from build123d import *

# Parameters (mm, degrees)
SALIENTE_EXTRUIR1_DEPTH = 1.5
CROQUIS2_W              = 25
CROQUIS2_H              = 3.1
CORTAR_EXTRUIR1_DEPTH   = 10


with BuildPart() as part:
    # Croquis1 → Saliente-Extruir1 (new, symmetric)
    with BuildSketch(Plane.XY):
        Polygon((-31.9, -27), (-31.9, -45), (-21, -45), (-21, -41.9), (-7, -41.9), (-7, -45), (7, -45), (7, -41.9), (21, -41.9), (21, -45), (31.9, -45), (31.9, -27), (35, -27), (35, -9), (31.9, -9), (31.9, 9), (35, 9), (35, 27), (31.9, 27), (31.9, 45), (21, 45), (21, 41.9), (7, 41.9), (7, 45), (-7, 45), (-7, 41.9), (-21, 41.9), (-21, 45), (-31.9, 45), (-31.9, 27), (-35, 27), (-35, 9), (-31.9, 9), (-31.9, -9), (-35, -9), (-35, -27), align=None)
    extrude(amount=SALIENTE_EXTRUIR1_DEPTH, both=True)

    # Croquis2 → Cortar-Extruir1 (cut)
    with BuildSketch(Plane(origin=(0, 0, -1.5), x_dir=(-1, 0, 0), z_dir=(0, 0, -1))):
        with Locations((0, -25.45)):
            Rectangle(CROQUIS2_W, CROQUIS2_H)
    extrude(amount=-CORTAR_EXTRUIR1_DEPTH, mode=Mode.SUBTRACT)


solid = part.part
Input: part model. Units: mm. Frame: model coordinates. A direction names the side the tool comes from. Round coordinates to 2 decimals unless told otherwise and drop trailing zeros. Write each loop counter-clockwise with the first axis right and the second up, starting at its lowest first coordinate (ties: lowest second). Pieces come first, ordered by that corner, then holes.
1) Cut plane C-C (y = 31). Return the cut outline in (x, z).
2) Cut plane B-B (y = -26). Return the cut outline in (x, z), then the cut area to 3 significant figures.
3) Ray query, L1, parallel to X at y = -25, z = 0.5; L2, parallel to Y at x = -11, z = 0.65; L3, parallel to Y at x = 1, z = 0.8. Return the intervals inside material, ascending.
4) Reachability of faces 4 (the flat face through (-31.9, -36, 0)), 5 (the flat face through (7, -43, 0)), 6 (the flat face through (-14, 41.9, 0)), 7 (the flat face through (-33, 27, 0)) from +Z, -Z, +X, -X, +Y, -Y: full face, straight path, thin tool, end or side. Return the list, or none.
5) Contact query for flat-ended pins moving along their axis: P1, Ø1.5, axis at y = -43.5, z = 0, coming from the +X side; P2, Ø0.9, axis at x = -14, z = -0.5, coming from the -Y side; P3, Ø1.5, axis at x = 33.5, z = 0, coming from the -Y side. Output: stop coordinate, or through.
6) Cut plane A-A (x = -6). Return the cut outline in (y, z).
7) Draft query along Y for faces 1 (the flat face through (21, -43, 0)), 2 (the flat face through (14, 41.9, 0)), 3 (the flat face through (-33, 9, 0)). Return one class per face: pulls with the +Y half, pulls with the -Y half, needs draft (parallel to the pull), parting line crosses it, or undercut.
Geometry says:
1. outline: (-31.9, -1.5) - (31.9, -1.5) - (31.9, 1.5) - (-31.9, 1.5) - close
2. outline: (-35, -1.5) - (-12.5, -1.5) - (-12.5, 1.5) - (-35, 1.5) - close; (12.5, -1.5) - (35, -1.5) - (35, 1.5) - (12.5, 1.5) - close
2. area: 135 mm2
3. L1: x = -35 to -12.5, 12.5 to 35
3. L2: y = -41.9 to -27, -23.9 to 41.9
3. L3: y = -45 to -27, -23.9 to 45
4. face 4: +Z, -Z, -X, -Y
4. face 5: +Z, -Z, -Y
4. face 6: +Z, -Z, +Y
4. face 7: +Z, -Z, -X, +Y
5. P1: stops at x = 31.9
5. P2: stops at y = -41.9
5. P3: stops at y = -27
6. outline: (-45, -1.5) - (-27, -1.5) - (-27, 1.5) - (-45, 1.5) - close; (-23.9, -1.5) - (45, -1.5) - (45, 1.5) - (-23.9, 1.5) - close
7. face 1: needs draft
7. face 2: pulls with the +Y half
7. face 3: undercut
